CAD build for the part. Positions are in the model's coordinates, mm. Give positions to 0.01 mm unless a question says otherwise; leave off trailing zeros. Loops run counter-clockwise (first coordinate to the right, second up) from the corner with the lowest first, then second, coordinate; pieces in that order, holes last.
Item 1: Saw through at C-C on z = 2.45. Give the cut face in (x, y) (1 decimal).
Item 2: Mould opens along X. For faces 1 (the flat face through (3.13, -7.89, 2.31)), 2 (the cylindrical face through (-2.106, -9.931, 1.91)), 3 (the cylindrical face through (0, -3, 5)), 4 (the flat face through (0, 0, 2)) say: released by +X, released by -X, zero draft, split by the parting line, or undercut.
Item 3: Probe probe 1 along Y at (x, z) = (0, 2.05); probe 2 along Y at (x, z) = (0.5, 3.5); probe 3 along Z at (x, y) = (2.75, -9.5). List the from-to ranges inside material, lowest first.
Item 4: Saw through at D-D on y = -3.75. Give the cut face in (x, z), plus the area to 3 significant figures.
Item 5: Saw through at A-A on x = 0. Give the cut face in (y, z), plus the area to 3 significant figures.
Item 6: Drop flat-ended pins along their axis: P1, Ø4.5, axis at x = 0, y = -8, coming from the -Z side; P2, Ø2, axis at y = -13.5, z = 1.5, coming from the +X side. Give the stop position or say it passes through.
Item 7: Saw through at B-B on y = -8. Give the cut face in (x, z).
from build123d import *

# Parameters (mm, degrees)
F1_DEPTH = 16
F2_R     = 2.8575
F3_DEPTH = 5.001


with BuildPart() as f1:
    # F0 (on Front) → F1 (new body)
    with BuildSketch(Plane.XZ):
        with BuildLine():
            ThreePointArc((-4.670489, 0.407251), (-4.701763, 0.142326), (-4.476139, 0))
            Line((-4.476139, 0), (4.476139, 0))
            ThreePointArc((4.476139, 0), (4.701763, 0.142326), (4.670489, 0.407251))
            Line((4.670489, 0.407251), (1.554805, 4.258008))
            ThreePointArc((1.554805, 4.258008), (0, 5), (-1.554805, 4.258008))
            Line((-1.554805, 4.258008), (-4.670489, 0.407251))
        make_face()
    extrude(amount=F1_DEPTH)

    # F2 (on face) → F3 (cut, through all)
    with BuildSketch(Plane(origin=(0, 0, 0), x_dir=(1, 0, 0), z_dir=(0, 0, -1))):
        with Locations((0, 8)):
            Circle(F2_R)
    extrude(amount=-F3_DEPTH, mode=Mode.SUBTRACT)


solid = f1.part
Results below:
1. outline: (-3, -16) - (3, -16) - (3, 0) - (-3, 0) - close; hole circle Ø5.7 at (0, -8)
2. face 1: released by +X
2. face 2: undercut
2. face 3: split by the parting line
2. face 4: zero draft
3. probe 1: y = -16 to -10.86, -5.14 to 0
3. probe 2: y = -16 to -10.81, -5.19 to 0
3. probe 3: z = 0 to 2.78
4. outline: (-4.67, 0.41) arc R0.25 ccw to (-4.48, 0) - (4.48, 0) arc R0.25 ccw to (4.67, 0.41) - (1.55, 4.26) arc R2 ccw to (-1.55, 4.26) - close
4. area: 29.4 mm2
5. outline: (-16, 0) - (-10.86, 0) - (-10.86, 5) - (-16, 5) - close; (-5.14, 0) - (0, 0) - (0, 5) - (-5.14, 5) - close
5. area: 51.4 mm2
6. P1: passes through
6. P2: stops at x = 4.6
7. outline: (-4.67, 0.41) arc R0.25 ccw to (-4.48, 0) - (-2.86, 0) - (-2.86, 2.65) - close; (2.86, 0) - (4.48, 0) arc R0.25 ccw to (4.67, 0.41) - (2.86, 2.65) - close
